Could you check a few things on this model? Use its own coordinates, in mm. Face numbers are marked on the shaded views. A direction names the side the tool comes from. Coordinates: 2 decimals unless noted, no trailing zeros. Loops run counter-clockwise (first coordinate to the right, second up) from the corner with the lowest first, then second, coordinate; pieces in that order, holes last. Notation, with made-up numbers: (37, -39) - (64, -39) arc R24 cw to (64, -2) - close; hole circle Ø4 at (77, 35). An arc over 180 degrees is marked (long way). Use CSV: the item, a comma, the result in double quotes.
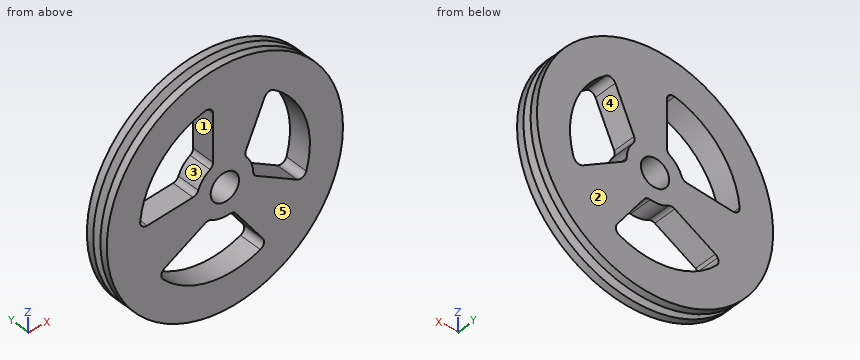
from build123d import *

# Parameters (mm, degrees)
F0_R     = 63.5
F0_R_2   = 7.62
F1_DEPTH = 6.35


with BuildPart() as f1:
    # F0 (on Front) → F1 (new body, symmetric)
    with BuildSketch(Plane.XZ):
        Circle(F0_R)
        with BuildLine():
            ThreePointArc((-33.697905, -27.295793), (-33.159597, -26.606146), (-32.464053, -26.075478))
            Line((-32.464053, -26.075478), (-10.594432, -13.449047))
            ThreePointArc((-10.594432, -13.449047), (-8.930055, -12.990774), (-7.25369, -13.403043))
            ThreePointArc((-7.25369, -13.403043), (-2.498289, -15.033834), (2.528965, -15.028704))
            ThreePointArc((2.528965, -15.028704), (4.391844, -15.235603), (5.866486, -16.392562))
            Line((5.866486, -16.392562), (20.419015, -36.426942))
            ThreePointArc((20.419015, -36.426942), (20.960921, -39.305626), (19.077861, -41.549412))
            ThreePointArc((19.077861, -41.549412), (-8.715152, -44.881672), (-33.241292, -31.390045))
            ThreePointArc((-33.241292, -31.390045), (-34.154471, -29.4193), (-33.697905, -27.295793))
        make_face(mode=Mode.SUBTRACT)
        with BuildLine():
            ThreePointArc((-45.521777, 4.252793), (-34.511093, 29.988379), (-10.56393, 44.482826))
            ThreePointArc((-10.56393, 44.482826), (-7.650549, 43.837984), (-6.35, 41.152434))
            Line((-6.35, 41.152434), (-6.35, 15.899571))
            ThreePointArc((-6.35, 15.899571), (-6.785313, 14.229042), (-7.980531, 12.983402))
            ThreePointArc((-7.980531, 12.983402), (-11.770537, 9.680499), (-14.279722, 5.324203))
            ThreePointArc((-14.279722, 5.324203), (-15.390341, 3.814353), (-17.129618, 3.115755))
            Line((-17.129618, 3.115755), (-41.756164, 0.530086))
            ThreePointArc((-41.756164, 0.530086), (-44.520131, 1.500123), (-45.521777, 4.252793))
        make_face(mode=Mode.SUBTRACT)
        Circle(F0_R_2, mode=Mode.SUBTRACT)
        with BuildLine():
            Line((11.263132, 13.276807), (21.33715, 35.896856))
            ThreePointArc((21.33715, 35.896856), (23.55921, 37.805503), (26.443915, 37.296618))
            ThreePointArc((26.443915, 37.296618), (43.226245, 14.893293), (43.805222, -13.092781))
            ThreePointArc((43.805222, -13.092781), (41.790083, -15.293422), (38.814053, -15.076956))
            Line((38.814053, -15.076956), (16.944432, -2.450524))
            ThreePointArc((16.944432, -2.450524), (15.715368, -1.238268), (15.234221, 0.419642))
            ThreePointArc((15.234221, 0.419642), (14.268826, 5.353335), (11.750756, 9.7045))
            ThreePointArc((11.750756, 9.7045), (10.998497, 11.42125), (11.263132, 13.276807))
        make_face(mode=Mode.SUBTRACT)
    extrude(amount=F1_DEPTH, both=True)

    # F2 (on Right) → F3 (revolve, cut)
    with BuildSketch(Plane.YZ):
        Polygon((-2.286, 63.5), (0, 54.61), (0, 63.5), align=None)
        Polygon((0, 63.5), (0, 54.61), (2.286, 63.5), align=None)
    revolve(axis=Axis((0, -4.296992, 0), (0, 1, 0)), mode=Mode.SUBTRACT)


solid = f1.part
(1) Will these pins go through, and if not, where does the flat tip stop? pin 1 (2 mm diameter, centred on x = 9.5, y = -4.5, fed in from +Z); pin 2 (5 mm diameter, centred on y = 0, z = 17.5, fed in from -X); pin 3 (4 mm diameter, centred on y = 4.5, z = -27, fed in from -X).
Computed:
pin 1,"stops at z = 62.93"
pin 2,"stops at x = -61.32"
pin 3,"stops at x = -58.37"
(2) Suppose I cut it at B-B (z = -6). State how many separate pieces and enclosed holes the cut face has, plus the area to 3 significant figures.
Computed:
separate pieces,"3"
enclosed holes,"0"
area,"1,160 mm²"
(3) Thinking about a two-plate mould opening in Z: for the marked faces 1, 2 and 3, which applies, +Z half, -Z half, draft (parallel to the pull), parting line (faces both ways), or undercut?
Computed:
face 1,"undercut"
face 2,"draft"
face 3,"undercut"
(4) Suppose I cut it at A-A (x = 0). Write out the boundary of the cut face in (y, z), plus the area to 3 significant figures.
Computed:
outline,"(-6.35, -63.5) - (-2.29, -63.5) - (0, -54.61) - (2.29, -63.5) - (6.35, -63.5) - (6.35, -45.72) - (-6.35, -45.72) - close; (-6.35, -15.24) - (6.35, -15.24) - (6.35, -7.62) - (-6.35, -7.62) - close; (-6.35, 7.62) - (6.35, 7.62) - (6.35, 63.5) - (2.29, 63.5) - (0, 54.61) - (-2.29, 63.5) - (-6.35, 63.5) - close"
area,"992 mm²"
(5) Please list where these lines run through material, in increasing order: line 1 (Z direction, x = 0, y = 3.75); line 2 (Z direction, x = 13.5, y = -3); line 3 (X direction, y = 2.5, z = 26).
Computed:
line 1,"z = -63.5 to -45.72, -15.24 to -7.62, 7.62 to 63.5"
line 2,"z = -62.05 to -43.68, -26.9 to 7.07, 18.3 to 62.05"
line 3,"x = -57.93 to -37.61, -6.35 to 16.93, 37.61 to 57.93"
(6) Which directions (+Z, -Z, +X, -X, +Y, -Y) give clear straight access to the entire face, cutting with the end or side of a thin tool? Please do the marked faces 4 and 5.
Computed:
face 4,"+Y, -Y"
face 5,"+Z, -Z, +X, -X, -Y"
